Could you check a few things on this model? Use its own coordinates, in mm. A direction names the side the tool comes from. Coordinates: 2 decimals unless noted, no trailing zeros. Write each loop counter-clockwise with the first axis right and the second up, starting at its lowest first coordinate (ties: lowest second). Pieces come first, ordered by that corner, then holes.
```python
from build123d import *

# Parameters (mm, degrees)
SKETCH1_R           = 15
BOSS_EXTRUDE1_DEPTH = 41
SKETCH2_R           = 10
BOSS_EXTRUDE2_DEPTH = 8.5
BOSS_EXTRUDE3_START = 5.5
SKETCH3_R           = 10
BOSS_EXTRUDE3_DEPTH = 5.5
SKETCH4_R           = 10
BOSS_EXTRUDE4_DEPTH = 10
BOSS_EXTRUDE5_START = 10
SKETCH5_R           = 10
BOSS_EXTRUDE5_DEPTH = 10


with BuildPart() as part:
    # Sketch1 → Boss-Extrude1 (new body)
    with BuildSketch(Plane.XY):
        Circle(SKETCH1_R)
    extrude(amount=BOSS_EXTRUDE1_DEPTH)

    # Sketch2 → Boss-Extrude2 (add)
    with BuildSketch(Plane.XY.offset(41)):
        Circle(SKETCH2_R)
    extrude(amount=BOSS_EXTRUDE2_DEPTH)

    # Sketch3 → Boss-Extrude3 (add)
    with BuildSketch(Plane(origin=(0, 0, 0), x_dir=(-1, 0, 0), z_dir=(0, 0, -1)).offset(BOSS_EXTRUDE3_START)):
        with Locations(Location((0, 0, 0), (0, 0, 180))):
            Circle(SKETCH3_R)
    extrude(amount=-BOSS_EXTRUDE3_DEPTH)

    # Sketch4 → Boss-Extrude4 (add)
    with BuildSketch(Plane.XY.offset(49.5)):
        Circle(SKETCH4_R)
    extrude(amount=BOSS_EXTRUDE4_DEPTH)

    # Sketch5 → Boss-Extrude5 (add)
    with BuildSketch(Plane(origin=(0, 0, -5.5), x_dir=(-1, 0, 0), z_dir=(0, 0, -1)).offset(BOSS_EXTRUDE5_START)):
        with Locations(Location((0, 0, 0), (0, 0, 180))):
            Circle(SKETCH5_R)
    extrude(amount=-BOSS_EXTRUDE5_DEPTH)


solid = part.part
```
Item 1: Which directions (+Z, -Z, +X, -X, +Y, -Y) give clear straight access to the entire face, cutting with the end or side of a thin tool? Please do faces 3 (the cylindrical face through (-2.17, -9.76, 50.12)), 4 (the cylindrical face through (-14.985, 0.66, 20.213)).
Item 2: If I drill on line 1 along Z through (x, y) = (13.25, 2.25); line 2 along X through (y, z) = (6.5, 55); line 3 along X through (y, z) = (-2.75, -7), over which ranges is the centre line in solid material (lowest first)?
Item 3: If we mould it in two halves opening along X, with no side actions, what happens to faces 1 (the cylindrical face through (-10, 0, -8)), 2 (the flat face through (3, -10, 0))? For each: released by +X, released by -X, zero draft, split by the parting line, or undercut.
Item 4: I want a section at A-A, the plane x = 0. List the corners of the cut face in (y, z) for me, then the cut area to 3 significant figures.
Item 5: I want a section at D-D, the plane y = -12. List the corners of the cut face in (x, z) for me.
Item 6: Will these pins go through, and if not, where does the flat tip stop? pin 1 Ø4 at (x, z) = (5.5, 37.5) entering from -Y; pin 2 Ø5 at (x, y) = (10.5, 11.5) entering from +Z; pin 3 Ø1 at (x, y) = (2, 10.5) entering from -Z.
Item 7: I want a section at C-C, the plane z = 20. List the corners of the cut face in (x, y) for me, then the cut area to 3 significant figures.
Taken from the geometry:
1. face 3: +Z
1. face 4: +Z, -Z
2. line 1: z = 0 to 41
2. line 2: x = -7.6 to 7.6
2. line 3: x = -9.61 to 9.61
3. face 1: split by the parting line
3. face 2: zero draft
4. outline: (-15, 0) - (-10, 0) - (-10, -15.5) - (10, -15.5) - (10, 0) - (15, 0) - (15, 41) - (10, 41) - (10, 59.5) - (-10, 59.5) - (-10, 41) - (-15, 41) - close
4. area: 1,910 mm2
5. outline: (-9, 0) - (9, 0) - (9, 41) - (-9, 41) - close
6. pin 1: stops at y = -14.59
6. pin 2: stops at z = 41
6. pin 3: stops at z = 0
7. outline: circle Ø30 at (0, 0)
7. area: 707 mm2
